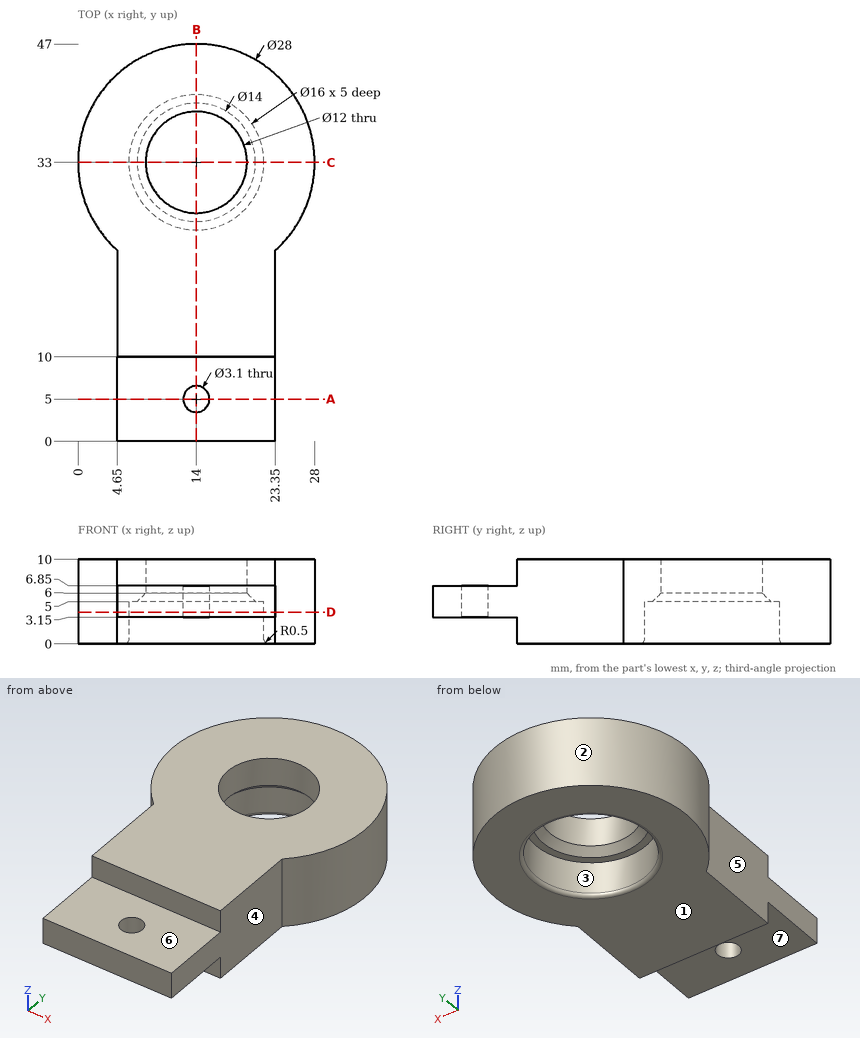
Check sheet for the drawn part. Datum: minimum x, y, z corner. Units: mm. A direction names the side the tool comes from. Give positions to 0.01 mm unless a question says otherwise; leave off trailing zeros. Order: outer loops, then holes, each group sorted by start corner. A loop starts at its lowest first (then second) coordinate and runs counter-clockwise, first axis right, second up.
1. Depth check by flat-ended pin: pin 1 (4 mm diameter, centred on y = 28.5, z = 1, fed in from -X) (3 decimals); pin 2 (1.6 mm diameter, centred on x = 15, z = 9, fed in from -Y); pin 3 (5 mm diameter, centred on x = 14, y = 5, fed in from -Z). Enter the tip coordinate at first touch or a pass-through.
Completed:
pin 1: stops at x = 0.225
pin 2: stops at y = 10
pin 3: stops at z = 3.15
2. Sectioned sample at D-D (z = 3.75). Record the boundary of the cut face in (x, y).
Completed:
outline: (4.65, 0) - (23.35, 0) - (23.35, 22.58) arc R14 ccw (long way) to (4.65, 22.58) - close; hole circle Ø16 at (14, 33); hole circle Ø3.1 at (14, 5)
3. Sectioned sample at C-C (y = 33). Record the boundary of the cut face in (x, z), then the cut area to 3 significant figures.
Completed:
outline: (0, 0) - (5.5, 0) arc R0.5 ccw to (6, 0.5) - (6, 5) - (7, 5) - (8, 6) - (8, 10) - (0, 10) - close; (20, 6) - (21, 5) - (22, 5) - (22, 0.5) arc R0.5 ccw to (22.5, 0) - (28, 0) - (28, 10) - (20, 10) - close
area: 139 mm2
4. Scan lines: line 1 (Y direction, x = 14, z = 4.5); line 2 (Y direction, x = 14, z = 1.5); line 3 (Y direction, x = 14, z = 5.25). Record each from-to range of solid material in increasing order.
Completed:
line 1: y = 0 to 3.45, 6.55 to 25, 41 to 47
line 2: y = 10 to 25, 41 to 47
line 3: y = 0 to 3.45, 6.55 to 26.25, 39.75 to 47
5. Access from +Z, -Z, +X, -X, +Y, -Y to the whole of each face (thin tool, end or side, straight path). Record for the marked faces 4, 5, 6 and 7.
Completed:
face 4: +Z, -Z, +X, -Y
face 5: +Z, -Z, -X, -Y
face 6: +Z, +X, -X, -Y
face 7: -Z, +X, -X, -Y
6. Draft check along Y on the marked faces 1, 2 and 3. Enter one of: pulls with the +Y half, pulls with the -Y half, needs draft (parallel to the pull), parting line crosses it, or undercut.
Completed:
face 1: needs draft
face 2: parting line crosses it
face 3: undercut
7. Sectioned sample at A-A (y = 5). Record the boundary of the cut face in (x, z), then the cut area to 3 significant figures.
Completed:
outline: (4.65, 3.15) - (12.45, 3.15) - (12.45, 6.85) - (4.65, 6.85) - close; (15.55, 3.15) - (23.35, 3.15) - (23.35, 6.85) - (15.55, 6.85) - close
area: 57.7 mm2
8. Sectioned sample at B-B (x = 14). State how many separate pieces and enclosed holes the cut face has, then the cut area to 3 significant figures.
Completed:
separate pieces: 3
enclosed holes: 0
area: 254 mm2
